Autodesk Inventor part; units mm, degrees
ref_plane "YZ Plane" through (0, 0, 0) normal (1, 0, 0) x (0, 1, 0)
ref_plane "XZ Plane" through (0, 0, 0) normal (0, 1, 0) x (-1, 0, 0)
ref_plane "XY Plane" through (0, 0, 0) normal (0, 0, 1) x (1, 0, 0)
sketch "Sketch1" plane through (0, 0, 0) normal (0, 0, 1) x (1, 0, 0)
  line L0 (-28, -34) -> (28, -34)
  line L1 (28, -34) -> (28, 34)
  line L2 (28, 34) -> (-28, 34)
  line L3 (-28, 34) -> (-28, -34)
  line L4 (-28, -34) -> (28, 34) construction
  line L5 (28, -34) -> (-28, 34) construction
  point P0 (0, 0)
  dimension "d0" = 56
  dimension "d1" = 68
extrude "Extrusion1" add sketch "Sketch1" along normal blind 12
sketch "Sketch2" plane through (28, -34, 0) normal (1, 0, 0) x (0, 0, -1)
  line L0 (0, 34) -> (-11.654, 34)
  line L1 (-11.654, 34) -> (-11.654, 11.5)
  line L2 (-11.654, 34) -> (-11.654, 56.5)
  circle A0 centre (-11.654, 11.5) radius 5.5
  circle A1 centre (-11.654, 56.5) radius 5.5
  dimension "d4" = 22.5
  dimension "d5" = 11
  dimension "d6" = 11
extrude "Extrusion2" cut sketch "Sketch2" against normal up to surface (56 mm away)
ref_plane "Work Plane1" through (25.5, -34, 0) normal (1, 0, 0) x (0, 0, -1)
sketch "Sketch3" plane through (25.5, -34, 0) normal (1, 0, 0) x (0, 0, -1)
  line L0 (-12, 51.0109) -> (-12, 16.9891)
  line L1 (-12, 61.9891) -> (-12, 68)
  line L2 (-12, 51.0109) -> (-12, 61.9891)
  line L3 (-12, 16.9891) -> (-12, 6.0109)
  circle A0 centre (-12, 11.5) radius 7.85
  circle A1 centre (-12, 56.5) radius 7.85
  point P0 (0, 34)
  dimension "d9" = 15.7
  dimension "d10" = 15.7
extrude "Extrusion3" cut sketch "Sketch3" against normal blind 24.5
ref_plane "Work Plane2" through (0, -34, 0) normal (1, 0, 0) x (0, 0, -1)
mirror "Mirror1" about plane through (0, -34, 0) normal (1, 0, 0) of "Extrusion3"
sketch "Sketch10" plane through (0, 0, 12) normal (0, 0, 1) x (1, 0, 0)
  line L0 (-8.9, 12.925) -> (8.9, 12.925)
  line L1 (8.9, 14.65) -> (8.9, -2.375)
  line L2 (8.9, -2.375) -> (-8.9, -2.375)
  line L3 (-8.9, -2.375) -> (-8.9, 12.925)
  line L4 (10.4, -4.375) -> (-10.4, -4.375)
  line L5 (10.4, 10.325) -> (10.4, -4.375)
  line L6 (-10.4, -4.375) -> (-10.4, 10.325)
  line L7 (-1, 14.65) -> (-25.5, 14.65)
  line L8 (-28, 17.0109) -> (-28, -17.0109)
  line L9 (28, -17.0109) -> (28, 17.0109)
  line L10 (-28, 10.325) -> (28, 10.325)
  line L11 (25.5, 14.65) -> (1, 14.65)
  line L12 (-1, -15.073) -> (1, -15.073)
  line L13 (0, -15.073) -> (0, -10.325)
  line L14 (28, -10.325) -> (-28, -10.325)
  line L15 (-15, -13.999) -> (15, -13.999)
  line L16 (15, -13.999) -> (15, -11.399)
  line L17 (15, -11.399) -> (-15, -11.399)
  line L18 (-15, -11.399) -> (-15, -13.999)
  line L19 (-15, -13.999) -> (15, -11.399) construction
  line L20 (15, -13.999) -> (-15, -11.399) construction
  line L21 (1, -14.65) -> (25.5, -14.65)
  point P0 (0, 0)
  point P1 (-28, 6.925)
  point P2 (28, 4.325)
  point P3 (21.4, 10.325)
  point P4 (0, -12.699)
  dimension "d82" = 2
  dimension "d83" = 1.5
  dimension "d84" = 1.5
  dimension "d105" = 15.3
  dimension "d116" = 2.6
  dimension "d117" = 30
  dimension "d152" = 0.651
extrude "Extrusion9" cut sketch "Sketch10" against normal up to surface (12 mm away) contours L17 L16 L15 L13 | L13 L15 L18 L17 | L0 L1 L10 L3 | L10 L1 L2 L3
sketch "Sketch12" plane through (0, 0, 12) normal (0, 0, 1) x (1, 0, 0)
  line L0 (-28, 10.325) -> (28, 10.325)
  line L1 (-10.4, 10.325) -> (-8.9, 10.325)
  line L2 (-8.9, 12.925) -> (-8.9, -2.375)
  line L3 (-1, 14.65) -> (-25.5, 14.65)
  line L4 (-8.9, 14.65) -> (-8.9, 10.325)
  line L5 (-8.9, 12.4875) -> (-13.55, 12.4875) construction
  circle A0 centre (-13.55, 12.4875) radius 1.65
  line L6 (28, -17.0109) -> (28, 17.0109) construction
  line L7 (28, 5.325) -> (21.4, 5.325) construction
  line L8 (21.4, 5.325) -> (21.4, 14.65) construction
  line L9 (21.4, 14.65) -> (28, 14.65) construction
  line L10 (28, 14.65) -> (28, 5.325) construction
  line L11 (21.4, 5.825) -> (21.4, 10.325) construction
  line L12 (25.5, 14.65) -> (1, 14.65)
  line L13 (21.4, 14.65) -> (28, 5.325) construction
  circle A1 centre (24.7, 9.9875) radius 1.65
  line L14 (-28, -34) -> (28, -34)
  line L15 (0, -34) -> (0, 34)
  circle A2 centre (13.55, 12.4875) radius 1.65
  line L16 (-15, -11.399) -> (-15, -13.999)
  line L17 (-15, -12.699) -> (-19.65, -12.699) construction
  circle A3 centre (-19.65, -12.699) radius 1.65
  circle A4 centre (19.65, -12.699) radius 1.65
  line L18 (-28, 7.925) -> (-18, 7.925) construction
  line L19 (-18, 7.925) -> (-18, 14.65) construction
  line L20 (-18, 14.65) -> (-28, 14.65) construction
  line L21 (-28, 14.65) -> (-28, 7.925) construction
  line L22 (-18, 10.325) -> (-18, 8.425) construction
  line L23 (-28, 14.65) -> (-18, 7.925) construction
  circle A5 centre (-23, 11.2875) radius 1.65
  line L24 (-28, 30.85) -> (28, 30.85) construction
  circle A6 centre (0, 32.5) radius 1.65
  line L25 (-25.5, 30.35) -> (-1, 30.35)
  line L26 (28, -34) -> (28, 34)
  line L27 (28, 0) -> (-28, 0)
  line L28 (-28, -30.85) -> (28, -30.85) construction
  circle A7 centre (0, -32.5) radius 1.65
  point P0 (0, 0)
  dimension "d118" = 4.65
  dimension "d119" = 3.3
  dimension "d121" = 3.3
  dimension "d122" = 4.65
  dimension "d123" = 3.3
  dimension "d124" = 3.3
  dimension "d125" = 3.3
  dimension "d126" = 0.5
extrude "Extrusion11" cut sketch "Sketch12" against normal up to surface (12 mm away) contours A6 | A5 L0 | L0 A5 | A1 L0 | L0 A1 | A7 L14 L15 | L15 L14 A7 | L14 A7 | A0 | A2 | A3 | A4
sketch "Sketch13" plane through (0, 0, 0) normal (0, 0, -1) x (-1, 0, 0)
  line L0 (3.4064, 38.1506) -> (5.8027, 34)
  line L1 (-5.8027, 34) -> (-3.4064, 38.1506)
  line L2 (-3.4064, 38.1506) -> (3.4064, 38.1506)
  line L3 (0, 34) -> (0, 32.2506)
  line L4 (-28, 34) -> (28, 34)
  line L5 (-28, 34) -> (28, 34)
  line L6 (-5.8027, 34) -> (5.8027, 34)
  line L7 (-28, -34) -> (-28, 34)
  line L8 (-28, 0) -> (28, 0)
  circle A0 centre (-24.7, 9.9875) radius 1.65
  line L9 (-29.7, 12.8743) -> (-24.7, 15.761)
  line L10 (-24.7, 15.761) -> (-19.7, 12.8743)
  line L11 (-19.7, 12.8743) -> (-19.7, 7.1007)
  line L12 (-19.7, 7.1007) -> (-24.7, 4.214)
  line L13 (-24.7, 4.214) -> (-29.7, 7.1007)
  line L14 (-29.7, 7.1007) -> (-29.7, 12.8743)
  line L15 (-28, 13.8557) -> (-28, 6.1193)
  circle A1 centre (0, -32.5) radius 1.65
  line L16 (-2.189, -36.2915) -> (-3.512, -34)
  line L17 (3.512, -34) -> (2.189, -36.2915)
  line L18 (2.189, -36.2915) -> (-2.189, -36.2915)
  line L19 (28, -34) -> (-28, -34)
  line L20 (-3.512, -34) -> (3.512, -34)
  point P0 (0, 0)
  dimension "d131" = 1.7494
  dimension "d142" = 10
extrude "Extrusion12" add sketch "Sketch13" against normal up to surface (12 mm away) contours L19 A1 L17 L18 L16 | L7 L13 L14 L9 | L0 L4 L1 L2 | L19 A1 picked at (-0.1173, -34.0374)
sketch "Sketch14" plane through (0, 0, 0) normal (0, 0, -1) x (-1, 0, 0)
  circle A0 centre (0, 32.5) radius 1.65
  line L0 (-1.65, 32.5) -> (1.65, 32.5) construction
  line L1 (1.7321, 35.5) -> (3.4641, 32.5)
  line L2 (3.4641, 32.5) -> (1.7321, 29.5)
  line L3 (1.7321, 29.5) -> (-1.7321, 29.5)
  line L4 (-1.7321, 29.5) -> (-3.4641, 32.5)
  line L5 (-3.4641, 32.5) -> (-1.7321, 35.5)
  line L6 (-1.7321, 35.5) -> (1.7321, 35.5)
  circle A1 centre (23, 11.2875) radius 1.65
  line L7 (26, 9.5554) -> (23, 7.8234)
  line L8 (23, 7.8234) -> (20, 9.5554)
  line L9 (20, 9.5554) -> (20, 13.0196)
  line L10 (20, 13.0196) -> (23, 14.7516)
  line L11 (23, 14.7516) -> (26, 13.0196)
  line L12 (26, 13.0196) -> (26, 9.5554)
  circle A2 centre (-24.7, 9.9875) radius 1.65
  line L13 (-27.7, 11.7196) -> (-24.7, 13.4516)
  line L14 (-24.7, 13.4516) -> (-21.7, 11.7196)
  line L15 (-21.7, 11.7196) -> (-21.7, 8.2554)
  line L16 (-21.7, 8.2554) -> (-24.7, 6.5234)
  line L17 (-24.7, 6.5234) -> (-27.7, 8.2554)
  line L18 (-27.7, 8.2554) -> (-27.7, 11.7196)
  circle A3 centre (0, -32.5) radius 1.65
  line L19 (1.7321, -29.5) -> (3.4641, -32.5)
  line L20 (3.4641, -32.5) -> (1.7321, -35.5)
  line L21 (1.7321, -35.5) -> (-1.7321, -35.5)
  line L22 (-1.7321, -35.5) -> (-3.4641, -32.5)
  line L23 (-3.4641, -32.5) -> (-1.7321, -29.5)
  line L24 (-1.7321, -29.5) -> (1.7321, -29.5)
  point P0 (0, 0)
  dimension "d138" = 6
  dimension "d139" = 6
  dimension "d140" = 6
  dimension "d141" = 6
extrude "Extrusion13" cut sketch "Sketch14" against normal blind 3.1
properties part number "custom"
Here's how the part is built. I have some questions about the finished solid (model axes, mm). A direction names the side the tool comes from. Coordinates: 2 decimals unless noted, no trailing zeros. Order: outer loops, then holes, each group sorted by start corner. A loop starts at its lowest first (then second) coordinate and runs counter-clockwise, first axis right, second up.
1) I need wall thicknesses on line 1 (Y direction, x = -6.5, z = 4) (3 decimals); line 2 (X direction, y = -28.5, z = 7); line 3 (Y direction, x = 9, z = 1.75). Which ranges of each line are inside material? Lowest first, please.
2) Imagine slicing it at A-A on x = 19.65. List the corners of the cut face in (y, z) for me, and give its area (3 significant figures).
3) Which directions (+Z, -Z, +X, -X, +Y, -Y) give clear straight access to the entire face, cutting with the end or side of a thin tool? Please do faces 1 (the face through (28, 24, 5)), 2 (the face through (-1, 34, 3.1)), 3 (the face through (-17, 34, 6)), 4 (the face through (25.5, -21, 6)), 5 (the face through (8.9, 5, 6)).
4) We'd pull the mould along X, two halves only. Please class faces 6 (the face through (1, -21, 6)), 7 (the face through (0, -36.292, 6)), 8 (the face through (0, 29.5, 2)), 9 (the face through (28.838, 6.603, 5.916)): +X half, -X half, draft (parallel to the pull), parting line (faces both ways), or undercut.
5) Will these pins go through, and if not, where does the flat tip stop? pin 1 (6 mm diameter, centred on x = 14, z = 9.5, fed in from +Y); pin 2 (4 mm diameter, centred on x = 10, z = 10.5, fed in from -Y); pin 3 (6 mm diameter, centred on y = 27, z = 3.5, fed in from +X).
6) Imagine slicing it at D-D on y = 22.5. List the corners of the cut face in (x, z) for me.
7) Imagine slicing it at B-B on y = -1. List the corners of the cut face in (x, z) for me.
8) Imagine slicing it at C-C on x = 13.55. List the corners of the cut face in (y, z) for me.
Response values:
1. line 1: y = -34 to -13.999, -11.399 to -2.375, 12.925 to 34
1. line 2: x = -28 to -25.5, -1 to 1, 25.5 to 28
1. line 3: y = -34 to -14, -11.4 to 34
2. outline: (-34, 0) - (-14.35, 0) - (-14.35, 12) - (-14.65, 12) arc R7.85 cw to (-30.35, 12) - (-34, 12) - close; (-11.05, 0) - (34, 0) - (34, 12) - (30.35, 12) arc R7.85 cw to (14.65, 12) - (-11.05, 12) - close
2. area: 583 mm2
3. face 1: +Z, -Z, +X, +Y
3. face 2: -Z
3. face 3: +Z, -Z, -X, +Y
3. face 4: +Z
3. face 5: +Z, -Z
4. face 6: undercut
4. face 7: draft
4. face 8: undercut
4. face 9: +X half
5. pin 1: stops at y = 34
5. pin 2: stops at y = -34
5. pin 3: stops at x = 28
6. outline: (-28, 0) - (28, 0) - (28, 6.15) - (25.5, 6.15) - (25.5, 4.15) - (1, 4.15) - (1, 6.15) - (-1, 6.15) - (-1, 4.15) - (-25.5, 4.15) - (-25.5, 6.15) - (-28, 6.15) - close
7. outline: (-28, 0) - (-8.9, 0) - (-8.9, 12) - (-28, 12) - close; (8.9, 0) - (28, 0) - (28, 12) - (8.9, 12) - close
8. outline: (-34, 0) - (-14, 0) - (-14, 12) - (-14.65, 12) arc R7.85 cw to (-30.35, 12) - (-34, 12) - close; (-11.4, 0) - (10.84, 0) - (10.84, 12) - (-11.4, 12) - close; (14.14, 0) - (34, 0) - (34, 12) - (30.35, 12) arc R7.85 cw to (14.65, 12) - (14.14, 12) - close
